CAD build for the part. Positions are in the model's coordinates, mm. A direction names the side the tool comes from. Give positions to 0.01 mm unless a question says otherwise; leave off trailing zeros. Write each loop counter-clockwise with the first axis right and the second up, starting at its lowest first coordinate (ties: lowest second). Pieces come first, ordered by that corner, then holes. Notation, with made-up numbers: (60.25, 45.25) -> (92.25, 45.25) arc R34 cw to (92.25, 80.25) -> close; hole circle Ø3 at (3.5, -12). An arc over 180 degrees is marked (long way). Answer as a JSON object with one key per item and string values.
```python
from build123d import *

# Parameters (mm, degrees)
F0_R      = 12.9
F1_DEPTH  = 3
F2_R      = 1.75
F3_DEPTH  = 3.001
F4_R      = 2.65
F5_DEPTH  = 12
F6_R      = 2.65
F7_DEPTH  = 12
F8_R      = 2.65
F9_DEPTH  = 12
F10_R     = 2.65
F11_DEPTH = 12
F12_R     = 2.65
F13_DEPTH = 12
F14_R     = 2.65
F15_DEPTH = 12


with BuildPart() as f1:
    # F0 (on Top) → F1 (new body)
    with BuildSketch(Plane.XY):
        Polygon((16.0075136901, 22.7174561645), (11.25, 26.956246243), (11.25, 31.956246243), (6.25, 31.956246243), (6.25, 26.956246243), (-6.25, 26.956246243), (-6.25, 31.956246243), (-11.25, 31.956246243), (-11.25, 26.956246243), (-16.0075136901, 22.7174561645), (-19.6075136901, 16.4820732572), (-20.8996567344, 10.2425505034), (-25.2297837534, 7.7425505034), (-22.7297837534, 3.4124234845), (-18.3996567344, 5.9124234845), (-12.1496567344, -4.9128940628), (-16.4797837534, -7.4128940628), (-13.9797837534, -11.7430210817), (-9.6496567344, -9.2430210817), (-3.6, -11.243753757), (3.6, -11.243753757), (9.6497229346, -9.2429064231), (13.9797837534, -11.7430210817), (16.4797837534, -7.4128940628), (12.1496567344, -4.9128940628), (18.3996567344, 5.9124234845), (22.7297837534, 3.4124234845), (25.2297837534, 7.7425505034), (20.8996567344, 10.2425505034), (19.6075136901, 16.4820732572), align=None)
        with Locations((0, 9.3591320669)):
            Circle(F0_R, mode=Mode.SUBTRACT)
    extrude(amount=F1_DEPTH)

    # F2 (on face) → F3 (cut, through all)
    with BuildSketch(Plane.XY.offset(3)):
        with Locations((-14.343412075, 17.5997647108)):
            Circle(F2_R)
        with Locations((14.343412075, 17.5997647108)):
            Circle(F2_R)
        with Locations((0, -7.243753757)):
            Circle(F2_R)
    extrude(amount=-F3_DEPTH, mode=Mode.SUBTRACT)

    # F4 (on face) → F5 (join)
    with BuildSketch(Plane(origin=(6.25, 0, 0), x_dir=(0, -1, 0), z_dir=(-1, 0, 0))):
        with Locations((-31.956246243, 1.5)):
            Circle(F4_R)
    extrude(amount=-F5_DEPTH)

    # F6 (on face) → F7 (join)
    with BuildSketch(Plane.YZ.offset(-6.25)):
        with Locations((31.956246243, 1.5)):
            Circle(F6_R)
    extrude(amount=-F7_DEPTH)

    # F8 (on face) → F9 (join)
    with BuildSketch(Plane(origin=(-7.1600686514, 12.4016026898, 0), x_dir=(0.8660254038, 0.5, 0), z_dir=(0.5, -0.8660254038, 0))):
        with Locations((-17.9783584107, 1.5)):
            Circle(F8_R)
    extrude(amount=-F9_DEPTH)

    # F10 (on face) → F11 (join)
    with BuildSketch(Plane(origin=(-0.9100686514, 1.5762851425, 0), x_dir=(-0.8660254038, -0.5, 0), z_dir=(-0.5, 0.8660254038, 0))):
        with Locations((17.9783584107, 1.5)):
            Circle(F10_R)
    extrude(amount=-F11_DEPTH)

    # F12 (on face) → F13 (join)
    with BuildSketch(Plane(origin=(0.9100686514, 1.5762851425, 0), x_dir=(-0.8660254038, 0.5, 0), z_dir=(0.5, 0.8660254038, 0))):
        with Locations((-17.9783584107, 1.5)):
            Circle(F12_R)
    extrude(amount=-F13_DEPTH)

    # F14 (on face) → F15 (join)
    with BuildSketch(Plane(origin=(7.1600686514, 12.4016026898, 0), x_dir=(0.8660254038, -0.5, 0), z_dir=(-0.5, -0.8660254038, 0))):
        with Locations((17.9783584107, 1.5)):
            Circle(F14_R)
    extrude(amount=-F15_DEPTH)


solid = f1.part
```
1) 3-axis set-ups, long thin cutter, end or side, ignore diameter. For faces 4 (the flat face through (-6.25, 31, 2)), 5 (the flat face through (13.66, 24.81, 1.48)), 6 (the flat face through (-15.32, 0.58, 1.48)): which of +Z, -Z, +X, -X, +Y, -Y reach the whole face in a straight line?
Model answer:
{"face 4": "+Z, -Z, +Y", "face 5": "+Z, -Z, +X", "face 6": "+Z, -Z"}
2) Slice it at A-A (x = 0). List the corners of the cut face in (y, z).
Model answer:
{"outline": "(-11.24, 0) -> (-8.99, 0) -> (-8.99, 3) -> (-11.24, 3) -> close; (-5.49, 0) -> (-3.54, 0) -> (-3.54, 3) -> (-5.49, 3) -> close; (22.26, 0) -> (26.96, 0) -> (26.96, 3) -> (22.26, 3) -> close"}
3) Pin check, flat tips, straight feed: pin 1 (5.5 mm diameter, centred on x = -14.34, y = 17.6, fed in from -Z); pin 2 (2.5 mm diameter, centred on y = 31, z = 2, fed in from -X); pin 3 (1.5 mm diameter, centred on x = 0, z = 2, fed in from -Y). Stop position of each tip, or through.
Model answer:
{"pin 1": "stops at z = 0", "pin 2": "stops at x = -18.25", "pin 3": "stops at y = -11.24"}
4) Wall check: probe 1 along X at (y, z) = (29.5, 1.2); probe 2 along Y at (x, z) = (15, 0.6); probe 3 along X at (y, z) = (28.5, 1.3). Give the ranges that are in metal, low to high.
Model answer:
{"probe 1": "x = -18.25 to -6.25, 6.25 to 18.25", "probe 2": "y = -14.96 to -6.56, 0.02 to 15.98, 19.22 to 23.62, 29.46 to 34.45", "probe 3": "x = -11.25 to -6.25, 6.25 to 11.25"}
5) Slice it at C-C (z = 1.5). State how many separate pieces and enclosed holes the cut face has, then the cut area to 3 significant figures.
Model answer:
{"separate pieces": "1", "enclosed holes": "4", "area": "1,110 mm2"}
6) Slice it at B-B (y = 20.5). List the corners of the cut face in (x, z).
Model answer:
{"outline": "(-17.29, 0) -> (-6.5, 0) -> (-6.5, 3) -> (-17.29, 3) -> close; (6.5, 0) -> (17.29, 0) -> (17.29, 3) -> (6.5, 3) -> close"}
7) Mould opens along X. For faces 1 (the cylindrical face through (-27.98, 7.21, 1.62)), 2 (the flat face through (-15.42, -6.8, 1.54)), 3 (the flat face through (28.7, 13.82, 1.54)) say: released by +X, released by -X, zero draft, split by the parting line, or undercut.
Model answer:
{"face 1": "undercut", "face 2": "released by -X", "face 3": "released by +X"}
